from build123d import *

# Parameters (mm, degrees)
SKETCH_W      = 200
SKETCH_H      = 200
PAD_DEPTH     = 10
SKETCH001_R   = 30
SKETCH001_R_2 = 10
SKETCH001_W   = 42.426406
SKETCH001_H   = 42.426406
SKETCH001_W_2 = 14.142136
SKETCH001_H_2 = 14.142136
POCKET_DEPTH  = 5


with BuildPart() as part:
    # Sketch → Pad (new body)
    with BuildSketch(Plane.XY):
        Rectangle(SKETCH_W, SKETCH_H)
    extrude(amount=PAD_DEPTH)

    # Sketch001 (on Face6 of Pad) → Pocket (cut)
    with BuildSketch(Plane.XY.offset(10)):
        with Locations((50, 50)):
            Circle(SKETCH001_R)
        with Locations((50, 50)):
            Circle(SKETCH001_R_2, mode=Mode.SUBTRACT)
        with BuildLine():
            add(Edge.make_bspline(
                [(-28.786797, -71.213203), (-10.415623, -52.84203), (-51.421015, -30.207812), (-92.426407, -7.573593), (-69.792188, -48.578985), (-47.15797, -89.584377), (-28.786797, -71.213203)],
                knots=[0, 0, 0, 2.094395, 2.094395, 4.18879, 4.18879, 6.283185, 6.283185, 6.283185], degree=2, weights=[1, 0.5, 1, 0.5, 1, 0.5, 1]))
        make_face()
        with BuildLine():
            add(Edge.make_bspline(
                [(-42.928932, -57.071068), (-36.805208, -50.947343), (-50.473672, -43.402604), (-64.142136, -35.857864), (-56.597396, -49.526328), (-49.052657, -63.194792), (-42.928932, -57.071068)],
                knots=[0, 0, 0, 2.094395, 2.094395, 4.18879, 4.18879, 6.283185, 6.283185, 6.283185], degree=2, weights=[1, 0.5, 1, 0.5, 1, 0.5, 1]))
        make_face(mode=Mode.SUBTRACT)
        Polygon((75.980762, -65), (50, -20), (24.019238, -65), align=None)
        Polygon((58.660254, -55), (50, -40), (41.339746, -55), align=None, mode=Mode.SUBTRACT)
        with Locations((-50, 50)):
            Rectangle(SKETCH001_W, SKETCH001_H)
        with Locations((-50, 50)):
            Rectangle(SKETCH001_W_2, SKETCH001_H_2, mode=Mode.SUBTRACT)
    extrude(amount=-POCKET_DEPTH, mode=Mode.SUBTRACT)


solid = part.part
Could you check a few things on this model? Use its own coordinates, in mm. A direction names the side the tool comes from. Coordinates: 2 decimals unless noted, no trailing zeros. Loops run counter-clockwise (first coordinate to the right, second up) from the corner with the lowest first, then second, coordinate; pieces in that order, holes last.
1. Imagine slicing it at A-A (z = 8.25). Give the number of separate pieces and of enclosed holes in the cut face, and give its area (3 significant figures).
2. For faces 1 (the face through (-1, 1, 10)), 2 (the face through (63, 50, 5)), which set-ups out of +Z, -Z, +X, -X, +Y, -Y let a thin tool reach every point of the face, with its end or its side?
3. Imagine slicing it at C-C (x = 45). Please give me the cut outline in (y, z).
4. Imagine slicing it at B-B (y = 50). Please give me the cut outline in (x, z), and give its area (3 significant figures).
5. We'd pull the mould along Y, two halves only. Please class faces 3 (the face through (50, -49, 10)), 4 (the face through (45.73, -47.395, 7.535)), 5 (the face through (-1, -100, 5)): released by +Y, released by -Y, zero draft, split by the parting line, or undercut.
6. For P1, Ø1, axis at x = -44.5, y = -38, coming from the +Z side, with a flat end and sliding along its axis, tell me the tip position at first contact or that it passes through.
7. I need wall thicknesses on L1, parallel to Y at x = 50, z = 6.55; L2, parallel to Y at x = 31.5, z = 9.75; L3, parallel to Y at x = -48.5, z = 8.75. Which ranges of each line are inside material? Lowest first, please.
Computed values:
1. separate pieces: 5
1. enclosed holes: 4
1. area: 33,600 mm2
2. face 1: +Z, +X, -X, +Y, -Y
2. face 2: +Z
3. outline: (-100, 0) - (100, 0) - (100, 10) - (79.58, 10) - (79.58, 5) - (58.66, 5) - (58.66, 10) - (41.34, 10) - (41.34, 5) - (20.42, 5) - (20.42, 10) - (-28.66, 10) - (-28.66, 5) - (-48.66, 5) - (-48.66, 10) - (-55, 10) - (-55, 5) - (-65, 5) - (-65, 10) - (-100, 10) - close
4. outline: (-100, 0) - (100, 0) - (100, 10) - (80, 10) - (80, 5) - (60, 5) - (60, 10) - (40, 10) - (40, 5) - (20, 5) - (20, 10) - (-28.79, 10) - (-28.79, 5) - (-42.93, 5) - (-42.93, 10) - (-57.07, 10) - (-57.07, 5) - (-71.21, 5) - (-71.21, 10) - (-100, 10) - close
4. area: 1,660 mm2
5. face 3: zero draft
5. face 4: undercut
5. face 5: released by -Y
6. P1: stops at z = 5
7. L1: y = -100 to -65, -55 to -40, -20 to 20, 40 to 60, 80 to 100
7. L2: y = -100 to -65, -52.04 to 26.38, 73.62 to 100
7. L3: y = -100 to -69.84, -57.11 to -44.69, -31.96 to 28.79, 42.93 to 57.07, 71.21 to 100
